Read the model definition and answer for the solid it produces. Units are mm, in the model's axes. Coordinates: 2 decimals unless noted, no trailing zeros. Write each loop counter-clockwise with the first axis right and the second up, starting at its lowest first coordinate (ties: lowest second). Pieces come first, ordered by that corner, then holes. Notation, with made-up numbers: M 6,47.25 L 52,47.25 A25 cw 52,71.25 Z; hole C 32,67.25 d4. An arc over 180 degrees is marked long. Use a Markdown table: item, result. Add a question column.
from build123d import *

# Parameters (mm, degrees)
BOSS_EXTRUDE1_DEPTH = 6.35
SKETCH2_W           = 19.05
SKETCH2_H           = 19.05
CUT_EXTRUDE1_DEPTH  = 715.888328692


with BuildPart() as part:
    # Sketch1 → Boss-Extrude1 (new body)
    with BuildSketch(Plane.XY):
        with BuildLine():
            Line((700, -53.219100704), (700, 0))
            Line((700, 0), (0, 0))
            Line((0, 0), (0, -97.708612477))
            ThreePointArc((0, -97.708612477), (0.615879968, -99.529593442), (2.210647783, -100.602903941))
            Line((2.210647783, -100.602903941), (164.612402034, -144.894291464))
            ThreePointArc((164.612402034, -144.894291464), (165.003554798, -144.97345543), (165.401754251, -145))
            Line((165.401754251, -145), (534.235017957, -145))
            ThreePointArc((534.235017957, -145), (534.976280341, -144.906979546), (535.671574349, -144.633686719))
            Line((535.671574349, -144.633686719), (698.436556392, -55.852787423))
            ThreePointArc((698.436556392, -55.852787423), (699.579696608, -54.750493995), (700, -53.219100704))
        make_face()
    extrude(amount=BOSS_EXTRUDE1_DEPTH)

    # Sketch2 → Cut-Extrude1 (cut, through all)
    with BuildSketch(Plane.XY.offset(6.35)):
        with Locations((9.525, -9.525)):
            Rectangle(SKETCH2_W, SKETCH2_H)
        with Locations((690.475, -9.525)):
            Rectangle(SKETCH2_W, SKETCH2_H)
    extrude(amount=-CUT_EXTRUDE1_DEPTH, mode=Mode.SUBTRACT)


solid = part.part
Item 1: Each of these flat-tipped pins is pushed along its axis until it touches: pin 1 (1.9 mm diameter, centred on x = 688.5, z = 3, fed in from +Y); pin 2 (3 mm diameter, centred on x = 540.5, z = 4, fed in from -Y). Where does it stop, or does it pass through?
Item 2: Find section B-B on x = 628.5. Give the vertices of the cut face in (y, z).
Item 3: Find section C-C on y = -88. Give the vertices of the cut face in (x, z), then the cut area to 3 significant figures.
Item 4: Find section A-A on z = 3.5. Give the vertices of the cut face in (x, y), then the cut area to 3 significant figures.
Item 5: Consider probe 1 along X at (y, z) = (-7.5, 2.75); probe 2 along X at (y, z) = (-69.5, 2.75); probe 3 along Y at (x, z) = (548.5, 4.5). Determine where each line is inside the solid, lowest interval first.
Geometry says:
| question | item | result |
|---|---|---|
| 1 | pin 1 | stops at y = -19.05 |
| 1 | pin 2 | stops at y = -142.82 |
| 2 | outline | M -94,0 L 0,0 L 0,6.35 L -94,6.35 Z |
| 3 | outline | M 0,0 L 639.5,0 L 639.5,6.35 L 0,6.35 Z |
| 3 | area | 4,060 mm2 |
| 4 | outline | M 0,-97.71 A3 ccw 2.21,-100.6 L 164.61,-144.89 A3 ccw 165.4,-145 L 534.24,-145 A3 ccw 535.67,-144.63 L 698.44,-55.85 A3 ccw 700,-53.22 L 700,-19.05 L 680.95,-19.05 L 680.95,0 L 19.05,0 L 19.05,-19.05 L 0,-19.05 Z |
| 4 | area | 89,600 mm2 |
| 5 | probe 1 | x = 19.05 to 680.95 |
| 5 | probe 2 | x = 0 to 673.42 |
| 5 | probe 3 | y = -137.64 to 0 |
